Drawing for the job (mm, zero at the part's lowest x, y, z). A direction names the side the tool comes from. Coordinates: 2 decimals unless noted, no trailing zeros. Write each loop counter-clockwise with the first axis right and the second up, starting at its lowest first coordinate (ties: lowest second). Pieces come first, ordered by that corner, then holes. Notation, with made-up numbers: (-12, -22) -> (-6, -22) arc R18 cw to (-6, -16) -> close; hole circle Ø6 at (47.25, 79). An arc over 180 degrees is marked (long way). Write item = value, one per line. Start each with the question number.
Q1. Band-saw the part on B-B, the plane y = 58.5. List the corners of the cut face in (x, z).
Q2. Tool access for the marked faces 1 and 2: list every direction of +Z, -Z, +X, -X, +Y, -Y with a clear straight run to the whole face (end or side of a thin tool).
Q3. Pin check, flat tips, straight feed: P1, Ø12, axis at x = 11, z = 26.5, coming from the -Y side; P2, Ø1, axis at x = 9.5, y = 20, coming from the -Z side (1 decimal); P3, Ø1, axis at y = 38, z = 26.5, coming from the -X side. Stop position of each tip, or through.
Q4. Probe line 1 (Y direction, x = 12.5, z = 21); line 2 (X direction, y = 34.5, z = 21.5) (1 decimal); line 3 (Z direction, x = 5.5, y = 38). List the from-to ranges inside material, lowest first.
Q5. Band-saw the part on A-A, the plane y = 47. List the corners of the cut face in (x, z) (1 decimal).
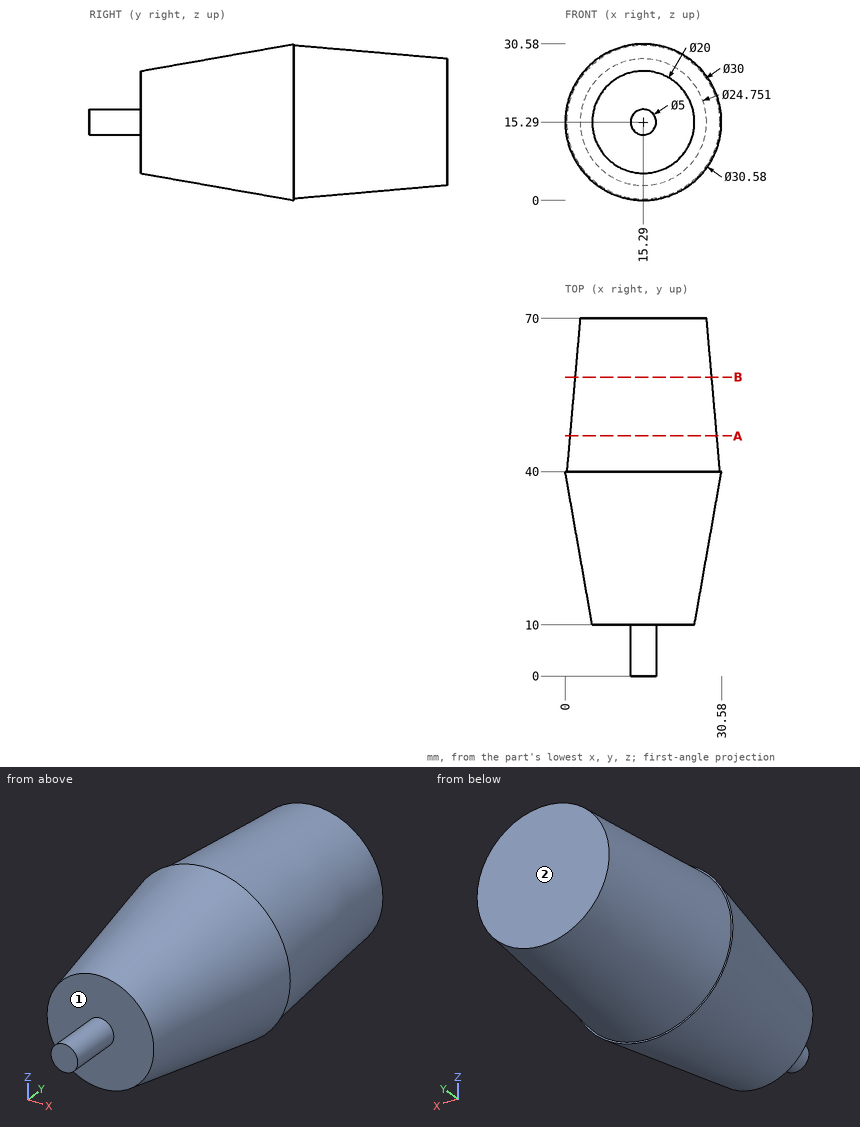
Ans:
q1.outline = circle Ø26.76 at (15.29, 15.29)
q2.face_1 = -Y
q2.face_2 = +Z, -Z, +X, -X, +Y
q3.P1 = 10
q3.P2 = 4.8
q3.P3 = 4.86
q4.line_1 = 10 to 70
q4.line_2 = 2.4 to 28.2
q4.line_3 = 4.01 to 26.57
q5.outline = circle Ø28.8 at (15.3, 15.3)
